from build123d import *

# Parameters (mm, degrees)
SKETCH248_R          = 3.9
PAD125_DEPTH         = 18.5
SKETCH249_R          = 1.4
PAD126_DEPTH         = 14.5
SKETCH252_R          = 2.75
POCKET034_DEPTH      = 0.001
POCKET034_DEPTH_BACK = 18.501


with BuildPart() as part:
    # Sketch248 → Pad125 (new body)
    with BuildSketch(Plane.XZ):
        Circle(SKETCH248_R)
    extrude(amount=PAD125_DEPTH)

    # Sketch249 → Pad126 (join)
    with BuildSketch(Plane.XZ.offset(2)):
        with Locations((-3, 0)):
            Circle(SKETCH249_R)
    extrude(amount=PAD126_DEPTH)

    # Sketch252 → Pocket034 (cut, two sides)
    with BuildSketch(Plane.XZ) as pocket034_sk:
        Circle(SKETCH252_R)
    extrude(amount=-POCKET034_DEPTH, mode=Mode.SUBTRACT)
    extrude(pocket034_sk.sketch, amount=POCKET034_DEPTH_BACK, mode=Mode.SUBTRACT)


with BuildPart() as part_1:
    # Body102 placement: moved
    add(part.part.moved(Location((0, 15, 0))))


solid = part_1.part
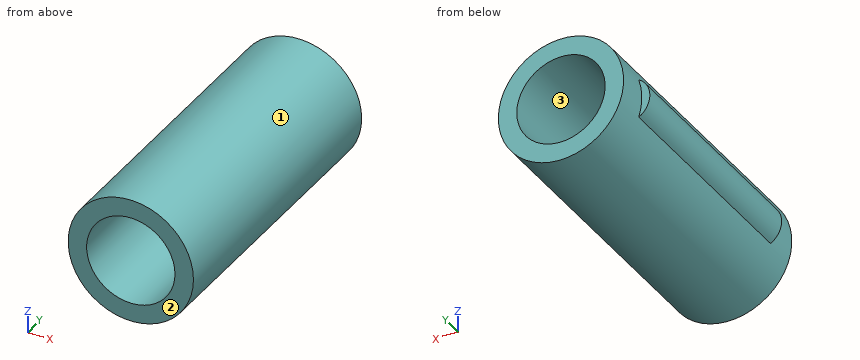
Design review of the part built by this model. Coordinates are the model's own, in mm. Face numbers are marked on the shaded views. Coordinates: 2 decimals unless noted, no trailing zeros. Loops run counter-clockwise (first coordinate to the right, second up) from the corner with the lowest first, then second, coordinate; pieces in that order, holes last. Notation, with made-up numbers: M -28.75,86 L 7.25,86 A21 cw 7.25,97 Z; hole C 3.25,-3 d8. An arc over 180 degrees is marked long. Use one line per item in the form item = value.
(1) Clearance check with a flat-ended pin moving along its axis: P1, Ø1.5, axis at x = 2, y = 0, coming from the -Z side. State where the tip first meets the part, or that it passes through.
Return value:
P1 = -3.69
(2) Consider section A-A (x = 0). Write out the cut boundary in (y, z), and give its area (4 significant figures).
Return value:
outline = M -3.5,-3.9 L 15,-3.9 L 15,-2.75 L -3.5,-2.75 Z; M -3.5,2.75 L 15,2.75 L 15,3.9 L -3.5,3.9 Z
area = 42.55 mm2
(3) Consider section B-B (z = 0). Write out the cut boundary in (x, y).
Return value:
outline = M -4.4,-1.5 L -3.9,-1.5 L -3.9,-3.5 L -2.75,-3.5 L -2.75,15 L -3.9,15 L -3.9,13 L -4.4,13 Z; M 2.75,-3.5 L 3.9,-3.5 L 3.9,15 L 2.75,15 Z
(4) Consider section C-C (y = 8.75). Write out the cut boundary in (x, z), and give its area (3 significant figures).
Return value:
outline = M -3.71,-1.21 A3.9 ccw long -3.71,1.21 A1.4 ccw Z; hole C 0,0 d5.5
area = 24.9 mm2
(5) Consider section D-D (z = 2). Write out the cut boundary in (x, y), and give its area (3 significant figures).
Return value:
outline = M -3.35,-3.5 L -1.89,-3.5 L -1.89,15 L -3.35,15 Z; M 1.89,-3.5 L 3.35,-3.5 L 3.35,15 L 1.89,15 Z
area = 54.0 mm2
(6) For line 1 along Z through (x, y) = (0, 12.5); line 2 along Z through (x, y) = (-1.75, 14); line 3 along X through (y, z) = (12.25, -1.25), list the stretches that pass through material, from the lowest coordinate up. Write a range as from..to.
Return value:
line_1 = -3.9..-2.75, 2.75..3.9
line_2 = -3.49..-2.12, 2.12..3.49
line_3 = -3.69..-2.45, 2.45..3.69
(7) Draft analysis for pull direction Z (two halves, no side actions). For the marked faces 1, 2 and 3, state which applies: pulls with the +Z half, pulls with the -Z half, needs draft (parallel to the pull), parting line crosses it, or undercut.
Return value:
face_1 = parting line crosses it
face_2 = needs draft
face_3 = undercut
